Design review of the part built by this model. Coordinates are the model's own, in mm. Face numbers are marked on the shaded views. A direction names the side the tool comes from. Round coordinates to 2 decimals unless told otherwise and drop trailing zeros. Write each loop counter-clockwise with the first axis right and the second up, starting at its lowest first coordinate (ties: lowest second). Pieces come first, ordered by that corner, then holes. Notation, with made-up numbers: (78, -39) - (119, -39) arc R19 cw to (119, -11) - close; hole circle Ø5 at (-33.75, 38.5). An arc over 180 degrees is marked (long way). Use one line per item in the form item = value.
```python
from build123d import *

# Parameters (mm, degrees)
SKETCH016_R        = 1.5
PAD011_DEPTH       = 10
SKETCH018_R        = 4
POCKET006005_DEPTH = 70.001
SKETCH019_W        = 2.985647
SKETCH019_H        = 2.199577
PAD012_DEPTH       = 24
SKETCH020_R        = 2.4
PAD013_DEPTH       = 6
SKETCH021_R        = 1.45
POCKET006006_DEPTH = 15.001


with BuildPart() as pocket006006:
    # Sketch016 → Pad011 (new body)
    with BuildSketch(Plane.XY.offset(2)):
        with BuildLine():
            ThreePointArc((-84.702782, 105.641821), (-80.035159, 112.152274), (-85.999598, 117.5))
            Line((-149.999599, 117.5), (-85.999598, 117.5))
            Line((-149.999599, -42.5), (-149.999599, 117.5))
            Line((-85.999599, -42.5), (-149.999599, -42.5))
            ThreePointArc((-85.999599, -42.5), (-80.035159, -37.152275), (-84.702781, -30.641821))
            Line((-125.999599, -21.5), (-84.702781, -30.641821))
            Line((-125.999599, 96.5), (-125.999599, -21.5))
            Line((-84.702782, 105.641821), (-125.999599, 96.5))
        make_face()
        with Locations((-85.999599, 111.5)):
            Circle(SKETCH016_R, mode=Mode.SUBTRACT)
        with Locations((-85.999599, -36.5)):
            Circle(SKETCH016_R, mode=Mode.SUBTRACT)
    extrude(amount=PAD011_DEPTH)

    # Sketch018 → Pocket006005 (cut, through all)
    with BuildSketch(Plane(origin=(-149.999599, 0, 2), x_dir=(0, -1, 0), z_dir=(-1, 0, 0))):
        with Locations((-75, -2)):
            Circle(SKETCH018_R)
        with Locations((0, -2)):
            Circle(SKETCH018_R)
    extrude(amount=-POCKET006005_DEPTH, mode=Mode.SUBTRACT)

    # Sketch019 → Pad012 (new body)
    with BuildSketch(Plane(origin=(-149.999599, 0, 2), x_dir=(0, -1, 0), z_dir=(-1, 0, 0))):
        with BuildLine():
            ThreePointArc((-3.614026, -3.714297), (1.858661, -5.541946), (3.464102, 0))
            Line((3.464102, 0), (9.949874, 0))
            ThreePointArc((9.949874, 0), (7.937413, -0.775141), (6.964912, -2.700001))
            ThreePointArc((-6.324555, -5), (1.193739, -8.897462), (6.964912, -2.700001))
            Line((-6.324555, -5), (-12.324555, -5))
            Line((-12.324555, -5), (-12.324555, -2))
            Line((-12.324555, -2), (-6.324546, -2))
            ThreePointArc((-3.614026, -3.714297), (-4.720978, -2.464543), (-6.324546, -2))
        make_face()
        with BuildLine():
            ThreePointArc((-78.464102, 0), (-76.858656, -5.541948), (-71.385969, -3.714287))
            ThreePointArc((-68.675445, -2), (-70.279013, -2.464538), (-71.385969, -3.714287))
            Line((-68.675445, -2), (-62.675445, -2))
            Line((-62.675445, -2), (-62.675445, -5))
            Line((-62.675445, -5), (-68.675445, -5))
            ThreePointArc((-81.964912, -2.700001), (-76.193739, -8.897462), (-68.675445, -5))
            ThreePointArc((-81.964912, -2.700001), (-82.937413, -0.775141), (-84.949874, 0))
            Line((-84.949874, 0), (-78.464102, 0))
        make_face()
        with Locations((-32.507176, -1.099789)):
            Rectangle(SKETCH019_W, SKETCH019_H)
    extrude(amount=-PAD012_DEPTH)

    # Sketch020 → Pad013 (new body)
    with BuildSketch(Plane(origin=(0, 34, 2), x_dir=(-1, 0, 0), z_dir=(0, 1, 0))):
        with BuildLine():
            Line((149.999599, 0), (125.999599, 0))
            Line((125.999599, 0), (125.999599, -9.999972))
            ThreePointArc((125.999599, -9.999972), (131.555682, -18.315281), (141.364245, -16.364245))
            Line((141.364245, -16.364245), (149.999599, -7.728891))
            Line((149.999599, -7.728891), (149.999599, 0))
        make_face()
        with Locations((135, -10)):
            Circle(SKETCH020_R, mode=Mode.SUBTRACT)
    extrude(amount=-PAD013_DEPTH)

    # Sketch021 → Pocket006006 (cut, through all)
    with BuildSketch(Plane(origin=(0, 0, -3), x_dir=(1, 0, 0), z_dir=(0, 0, -1))):
        with Locations((-145.999599, -9.324555)):
            Circle(SKETCH021_R)
        with Locations((-137.999599, -9.324555)):
            Circle(SKETCH021_R)
        with Locations((-129.999599, -9.324555)):
            Circle(SKETCH021_R)
        with Locations((-145.999599, -65.675445)):
            Circle(SKETCH021_R)
        with Locations((-137.999599, -65.675445)):
            Circle(SKETCH021_R)
        with Locations((-129.999599, -65.675445)):
            Circle(SKETCH021_R)
    extrude(amount=-POCKET006006_DEPTH, mode=Mode.SUBTRACT)


with BuildPart() as part_mirroring:
    # Part__Mirroring: instance of Pocket006006
    add(pocket006006.part.mirror(Plane(origin=(0, 0, 0), x_dir=(0, -1, 0), z_dir=(1, 0, 0))))


solid = part_mirroring.part
```
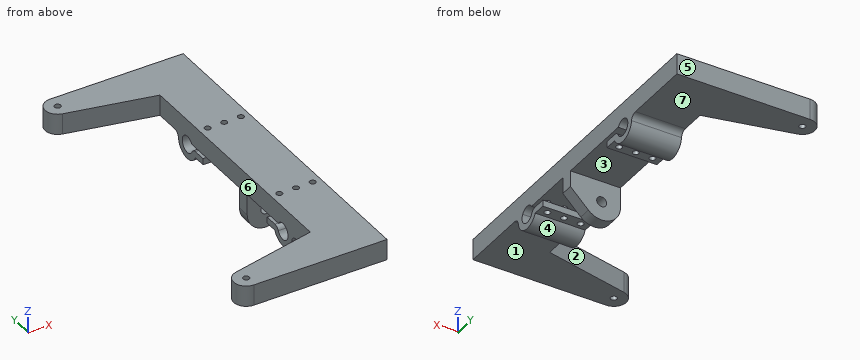
Q1. For P1, Ø4, axis at x = 135.5, y = 68.5, coming from the -Z side; P2, Ø3.5, axis at x = 137, z = -2, coming from the +Y side; P3, Ø8, axis at x = 136.5, z = -12, coming from the +Y side, all flat-tipped, find the tip position at first contact; note any pin that passes through.
Calculated:
P1 = -5.36
P2 = 82.05
P3 = 34
Q2. We need section C-C on y = 104. Write out the cut boundary in (x, z), then the cut area to 3 significant figures.
Calculated:
outline = (92.12, 2) - (150, 2) - (150, 12) - (92.12, 12) - close
area = 579 mm2
Q3. Machinability: for the marked faces 1, 2 and 3, which of the approach directions +Z, -Z, +X, -X, +Y, -Y give a long, thin tool a straight path to every point of the face, cutting with its end or side? Answer none if there is none.
Calculated:
face_1 = -Z, +X, -X, -Y
face_2 = +Z, -Z, -X
face_3 = +X, -X
Q4. To check wall thickness, follow line 1 along Y through (x, z) = (146.5, 4.5); line 2 along Y through (x, z) = (135, -5.5); line 3 along Y through (x, z) = (133, -2). State the ranges of each line that lie inside material, in increasing order. Write a range as from..to.
Calculated:
line_1 = -42.5..7.96, 10.69..64.31, 67.04..117.5
line_2 = -4.33..4.33, 28..34, 70.67..79.33
line_3 = -6.71..-3.46, 3.46..12.32, 28..34, 62.68..71.54, 78.46..81.71
Q5. Draft analysis for pull direction Y (two halves, no side actions). For the marked faces 4, 5, 6 and 7, state which applies: released by +Y, released by -Y, zero draft, split by the parting line, or undercut.
Calculated:
face_4 = undercut
face_5 = released by +Y
face_6 = undercut
face_7 = zero draft
Q6. We need section B-B on x = 119. Write out the cut boundary in (y, z).
Calculated:
outline = (-42.5, 2) - (-23.05, 2) - (-23.05, 12) - (-42.5, 12) - close; (98.05, 2) - (117.5, 2) - (117.5, 12) - (98.05, 12) - close
Q7. We need section A-A on y = 0. Write out the cut boundary in (x, z), then the cut area to 3 significant figures.
Calculated:
outline = (126, -7) - (150, -7) - (150, -4) - (126, -4) - close; (126, 4) - (150, 4) - (150, 12) - (126, 12) - close
area = 264 mm2
